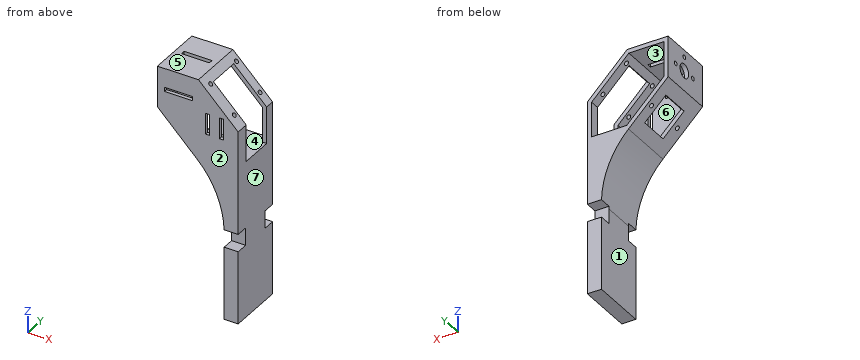
Autodesk Inventor part; units mm, degrees
ref_plane "YZ Plane" through (0, 0, 0) normal (1, 0, 0) x (0, 1, 0)
ref_plane "XZ Plane" through (0, 0, 0) normal (0, 1, 0) x (-1, 0, 0)
ref_plane "XY Plane" through (0, 0, 0) normal (0, 0, 1) x (1, 0, 0)
sketch "Sketch1" plane through (0, 0, 0) normal (0, 1, 0) x (-1, 0, 0)
  line L0 (10.6066, 0) -> (0, -10.6066)
  line L1 (0, -10.6066) -> (0, -20.6066)
  line L2 (0, -20.6066) -> (10, -20.6066)
  line L3 (10, -20.6066) -> (20.6066, -10)
  line L4 (20.6066, -10) -> (20.6066, 0)
  line L5 (20.6066, 0) -> (10.6066, 0)
  line L6 (21.8066, 1.2) -> (21.8066, -10.4971)
  line L7 (21.8066, -10.4971) -> (10.4971, -21.8066)
  line L8 (10.4971, -21.8066) -> (-1.2, -21.8066)
  line L9 (-1.2, -21.8066) -> (-1.2, -10.1095)
  line L10 (-1.2, -10.1095) -> (10.1095, 1.2)
  line L11 (10.1095, 1.2) -> (21.8066, 1.2)
  line L12 (-1.2, -21.8066) -> (-1.2, -40.3889)
  line L13 (-1.2, -40.3889) -> (2.8, -40.3889)
  arc A0 (10.4971, -21.8066) -> (2.8, -40.3889) centre (29.0794, -40.3889) ccw
  line L14 (4.8083, -4.1012) -> (5.5154, -4.8083) construction
  line L15 (5.5154, -4.8083) -> (13.9559, -4.8083) construction
  line L16 (5.5154, -4.8083) -> (5.5154, -15.0259) construction
  line L17 (-1.2, -40.3889) -> (2.8, -40.3889)
  line L18 (2.8, -40.3889) -> (2.8, -65.3889)
  line L19 (2.8, -65.3889) -> (-1.2, -65.3889)
  line L20 (-1.2, -65.3889) -> (-1.2, -40.3889)
  point P0 (0, 0)
  point P1 (4.4548, -4.4548)
  dimension "d0" = 135
  dimension "d2" = 15
  dimension "d3" = 10
  dimension "d4" = 10
  dimension "d5" = 10
  dimension "d6" = 1.2
  dimension "d29" = 4
  dimension "d44" = 1
  dimension "d45" = 0.5
  dimension "d52" = 25
extrude "Extrusion1" add sketch "Sketch1" along normal blind 1 contours L5 L4 L3 L2 L1 L0
extrude "Extrusion2" add sketch "Sketch1" along normal blind 16
sketch "Sketch2" plane through (1.2, 0, -10.1095) normal (0.7071, 0, 0.7071) x (0.7071, 0, -0.7071)
  line L0 (-15.9941, 0) -> (0, 0)
  line L1 (0, 0) -> (0, 16)
  line L2 (-15.9941, 16) -> (0, 16)
  line L3 (-15.9941, 0) -> (-15.9941, 16)
  line L4 (-13.2471, 13.25) -> (-3.7471, 13.25)
  line L5 (-3.7471, 13.25) -> (-3.7471, 3.75)
  line L6 (-3.7471, 3.75) -> (-13.2471, 3.75)
  line L7 (-13.2471, 3.75) -> (-13.2471, 13.25)
  circle A0 centre (-13.2471, 14.5) radius 0.6
  circle A1 centre (-3.7471, 14.5) radius 0.6
  circle A2 centre (-3.7471, 2.5) radius 0.6
  circle A3 centre (-13.2471, 2.5) radius 0.6
  point P0 (-7.9971, 0)
  point P1 (-8.4971, 13.25)
  point P2 (-7.9971, 16)
  point P3 (-13.2471, 8.5)
  point P4 (-15.9941, 8)
  point P5 (-8.4971, 0)
  point P6 (-8.4971, 0)
  point P7 (-8.4971, 0)
  dimension "d11" = 0.5
  dimension "d12" = 9.5
  dimension "d13" = 6
  dimension "d14" = 6
  dimension "d15" = 1.2
extrude "Extrusion3" cut sketch "Sketch2" against normal blind 2 contours L4 L5 L6 L7 | A0 | A1 | A2 | A3
sketch "Sketch3" plane through (1.2, 0, -10.1095) normal (1, 0, 0) x (0, 0, -1)
  line L0 (-9.3671, 13.25) -> (-2.6496, 13.25)
  line L1 (-2.6496, 3.75) -> (-9.3671, 3.75)
  line L2 (-2.6496, 3.75) -> (10.4971, 3.75)
  line L3 (10.4971, 3.75) -> (10.4971, 13.25)
  line L4 (10.4971, 13.25) -> (-2.6496, 13.25)
  line L5 (-2.6496, 13.25) -> (-2.6496, 3.75)
  line L6 (10.4971, 1) -> (10.4971, 16)
  line L7 (0, 16) -> (55.2794, 16)
  line L8 (55.2794, 0) -> (55.2794, 16)
  line L9 (0, 0) -> (55.2794, 0)
  line L10 (34.4971, 0) -> (29.4971, 0)
  line L11 (29.4971, 0) -> (29.4971, 3.5)
  line L12 (29.4971, 3.5) -> (34.4971, 3.5)
  line L13 (34.4971, 3.5) -> (34.4971, 0)
  line L14 (29.4971, 16) -> (34.4971, 16)
  line L15 (34.4971, 16) -> (34.4971, 12.5)
  line L16 (34.4971, 12.5) -> (29.4971, 12.5)
  line L17 (29.4971, 12.5) -> (29.4971, 16)
  point P0 (-10.1095, 0)
  point P1 (55.2794, 8)
  dimension "d59" = 5
  dimension "d60" = 9
  dimension "d66" = 20.7823
extrude "Extrusion4" cut sketch "Sketch3" against normal up to next
sketch "Sketch4" plane through (-21.8066, 0, -10.4971) normal (-0.7071, 0, -0.7071) x (-0.7071, 0, 0.7071)
  line L0 (-15.9941, 0) -> (0, 0)
  line L1 (0, 0) -> (0, 16)
  line L2 (-15.9941, 16) -> (0, 16)
  line L3 (-15.9941, 0) -> (-15.9941, 16)
  line L4 (-12.2471, 12.75) -> (-3.7471, 12.75)
  line L5 (-3.7471, 12.75) -> (-3.7471, 4.25)
  line L6 (-3.7471, 4.25) -> (-12.2471, 4.25)
  line L7 (-12.2471, 4.25) -> (-12.2471, 12.75)
  circle A0 centre (-7.9971, 14.5) radius 0.6
  circle A1 centre (-7.9971, 2.5) radius 0.6
  point P0 (-7.9971, 0)
  point P1 (-7.9971, 12.75)
  point P2 (-7.9971, 16)
  point P3 (0, 8)
  point P4 (-3.7471, 8.5)
  point P5 (-12.2471, 8.5)
  dimension "d21" = 0.5
  dimension "d22" = 8.5
  dimension "d23" = 6
  dimension "d24" = 6
  dimension "d25" = 1.2
extrude "Extrusion5" cut sketch "Sketch4" against normal blind 2 contours L4 L5 L6 L7 | A0 | A1
sketch "Sketch5" plane through (-21.8066, 0, -10.4971) normal (-1, 0, 0) x (0, 0, 1)
  line L0 (10.4971, 1) -> (10.4971, 16)
  circle A0 centre (5.6887, 8.5) radius 2
  circle A1 centre (5.6887, 12.5) radius 0.6
  circle A2 centre (5.6887, 4.5) radius 0.6
  circle A3 centre (9.6887, 8.5) radius 0.6
  point P0 (10.4971, 0)
  point P1 (10.4971, 8.5)
  point P2 (5.6887, 0)
  point P3 (5.6887, 0)
  point P4 (5.6887, 0)
  dimension "d30" = 4
  dimension "d31" = 1.2
  dimension "d32" = 4
  dimension "d33" = 4
  dimension "d34" = 4
extrude "Extrusion6" cut sketch "Sketch5" against normal blind 2
sketch "Sketch6" plane through (0, 0, 0) normal (0, -1, 0) x (1, 0, 0)
  line L0 (-21.8066, -6.8083) -> (-21.8066, -2.8083)
  line L1 (-11.8066, -7.4083) -> (-19.8066, -7.4083)
  line L2 (-19.8066, -7.4083) -> (-19.8066, -6.2083)
  line L3 (-19.8066, -6.2083) -> (-11.8066, -6.2083)
  line L4 (-11.8066, -6.2083) -> (-11.8066, -7.4083)
  line L5 (-11.8066, -3.4083) -> (-19.8066, -3.4083)
  line L6 (-19.8066, -3.4083) -> (-19.8066, -2.2083)
  line L7 (-19.8066, -2.2083) -> (-11.8066, -2.2083)
  line L8 (-11.8066, -2.2083) -> (-11.8066, -3.4083)
  line L9 (-15.8066, -6.2083) -> (-15.8066, -3.4083) construction
  line L10 (-5.5154, -4.8083) -> (-13.9559, -4.8083) construction
  line L11 (-5.5154, -4.8083) -> (-5.5154, -15.0259) construction
  line L12 (-8.1154, -13.8083) -> (-6.9154, -13.8083)
  line L13 (-6.9154, -13.8083) -> (-6.9154, -7.8083)
  line L14 (-6.9154, -7.8083) -> (-8.1154, -7.8083)
  line L15 (-8.1154, -7.8083) -> (-8.1154, -13.8083)
  line L16 (-4.1154, -13.8083) -> (-2.9154, -13.8083)
  line L17 (-2.9154, -13.8083) -> (-2.9154, -7.8083)
  line L18 (-2.9154, -7.8083) -> (-4.1154, -7.8083)
  line L19 (-4.1154, -7.8083) -> (-4.1154, -13.8083)
  line L20 (-4.1154, -10.8083) -> (-6.9154, -10.8083) construction
  line L21 (-11.8066, -5.4083) -> (-19.8066, -5.4083)
  line L22 (-19.8066, -5.4083) -> (-19.8066, -4.2083)
  line L23 (-19.8066, -4.2083) -> (-11.8066, -4.2083)
  line L24 (-11.8066, -4.2083) -> (-11.8066, -5.4083)
  line L25 (-5.6154, -7.8083) -> (-5.4154, -7.8083)
  line L26 (-5.4154, -7.8083) -> (-5.4154, -13.8083)
  line L27 (-5.4154, -13.8083) -> (-5.6154, -13.8083)
  line L28 (-5.6154, -13.8083) -> (-5.6154, -7.8083)
  point P0 (0, 0)
  point P1 (-21.8066, -4.8083)
  point P2 (-19.8066, -2.8083)
  point P3 (-19.8066, -6.8083)
  point P4 (-15.8066, -7.4083)
  point P5 (-15.8066, -4.8083)
  point P6 (-5.5154, -10.8083)
  point P7 (-3.5154, -13.8083)
  point P8 (-7.5154, -13.8083)
  point P9 (-19.8066, -4.8083)
  point P10 (-5.5154, -7.8083)
  dimension "d38" = 1.2
  dimension "d39" = 4
  dimension "d40" = 8
  dimension "d41" = 6
  dimension "d46" = 1.2
  dimension "d47" = 6
  dimension "d48" = 4
  dimension "d49" = 3
  dimension "d51" = 1.3
  dimension "d62" = 1.2
extrude "Extrusion7" cut sketch "Sketch6" against normal blind 25.4 contours L15 L14 L13 L12 | L19 L18 L17 L16 | L21 L22 L23 L24
sketch "Sketch7" plane through (-21.8066, 0, 1.2) normal (0, 0, 1) x (1, 0, 0)
  line L0 (2, 0) -> (10, 0)
  line L1 (0, 6.5) -> (0, 10.5)
  line L2 (2, 9.1) -> (10, 9.1)
  line L3 (10, 9.1) -> (10, 7.9)
  line L4 (10, 7.9) -> (2, 7.9)
  line L5 (2, 7.9) -> (2, 9.1)
  point P0 (21.8066, 0)
  point P1 (2, 8.5)
  point P2 (0, 8.5)
  dimension "d63" = 1.2
extrude "Extrusion8" cut sketch "Sketch7" against normal up to next
properties part number "tactic2 chassis1"
The listing builds one solid part. Answer for the finished solid, in the listing's coordinates (mm). Face numbers are marked on the shaded views. A direction names the side the tool comes from. Give positions to 0.01 mm unless a question says otherwise; leave off trailing zeros. Loops run counter-clockwise (first coordinate to the right, second up) from the corner with the lowest first, then second, coordinate; pieces in that order, holes last.
Item 1: Determine the mould class of the marked faces 4, 5, 6 and 7 for opening direction Z: +Z half, -Z half, draft (parallel to the pull), parting line (faces both ways), or undercut.
Derived:
face 4: undercut
face 5: +Z half
face 6: undercut
face 7: draft
Item 2: A cutting plane is placed at A-A (y = 8.5). Give the number of separate pieces and of enclosed holes in the cut face, then the cut area to 3 significant figures.
Derived:
separate pieces: 5
enclosed holes: 0
area: 254 mm2
Item 3: A tool of negligible diameter and unlimited length cuts with its end or side. For the marked faces 1, 2 and 3, from which of +Z, -Z, +X, -X, +Y, -Y can it reach the whole face along a straight path? Write none if from no direction.
Derived:
face 1: -Z, -X, +Y, -Y
face 2: +Z, -Z, +X, -X, -Y
face 3: +Y
Item 4: A cutting plane is placed at D-D (z = -46). Give the vertices of the cut face in (x, y), then the cut area to 3 significant figures.
Derived:
outline: (-2.8, 0) - (1.2, 0) - (1.2, 16) - (-2.8, 16) - close
area: 64.0 mm2
Item 5: A cutting plane is placed at B-B (x = -5.5). Give the vertices of the cut face in (y, z).
Derived:
outline: (0, -28.79) - (16, -28.79) - (16, -20.61) - (1, -20.61) - (1, -5.11) - (3.75, -5.11) - (3.75, -3.41) - (0, -3.41) - close; (13.25, -5.11) - (16, -5.11) - (16, -3.41) - (13.25, -3.41) - close
Item 6: A cutting plane is placed at C-C (z = -11.5). Give the vertices of the cut face in (x, y), then the cut area to 3 significant figures.
Derived:
outline: (-20.8, 0) - (-8.12, 0) - (-8.12, 1) - (-19.11, 1) - (-19.11, 16) - (-20.8, 16) - close; (-6.92, 0) - (-4.12, 0) - (-4.12, 1) - (-6.92, 1) - close; (-2.92, 0) - (1.2, 0) - (1.2, 3.75) - (0, 3.75) - (0, 1) - (-2.92, 1) - close; (0, 13.25) - (1.2, 13.25) - (1.2, 16) - (0, 16) - close
area: 51.7 mm2
Item 7: Find the intervals of material crossed by line 1 along Z through (x, y) = (-1.25, 14.5); line 2 along Z through (x, y) = (-0.25, 13.5); line 3 along X through (y, z) = (13.5, -62), in increasing order.
Derived:
line 1: z = -65.39 to -44.61, -39.61 to -20.61, -9.36 to -8.11
line 2: z = -65.39 to -44.61, -39.61 to -20.61, -10.36 to -8.66
line 3: x = -2.8 to 1.2
Item 8: Each of these flat-tipped pins is pushed along its axis until it touches: pin 1 Ø3.5 at (x, y) = (-6.5, 12) entering from +Z; pin 2 Ø4 at (x, y) = (0, 1.5) entering from +Z; pin 3 Ø1 at (x, y) = (-18.5, 14.5) entering from -Z; pin 4 Ø1.1 at (y, z) = (4.5, -4.81) entering from +X. Where does it stop, or does it pass through?
Derived:
pin 1: stops at z = -0.66
pin 2: stops at z = -6.91
pin 3: stops at z = -14.3
pin 4: passes through
